The model under review builds one solid part; all positions refer to its coordinate system, in mm. Face numbers are marked on the shaded views. A direction names the side the tool comes from. Round coordinates to 2 decimals unless told otherwise and drop trailing zeros. Order: outer loops, then holes, each group sorted by start corner. A loop starts at its lowest first (then second) coordinate and runs counter-clockwise, first axis right, second up. Notation, with made-up numbers: M 27,-21.5 L 75,-21.5 A21 ccw 75,13.5 Z; hole C -3.75,85 d1. An arc over 180 degrees is marked long. Answer as a JSON object with one key per item and string values. Group by question number.
1. Add section D-D on y = -29.5. State the section outline as (x, z) points, and give its area (3 significant figures).
2. Clearance check with flat-ended pins moving along their axes: P1, Ø1, axis at y = -17, z = 6, coming from the +X side; P2, Ø16, axis at x = 0.5, y = -4, coming from the +Z side; P3, Ø1.5, axis at y = -32.5, z = 1, coming from the -X side; P4, Ø10, axis at x = 11, y = 0.5, coming from the -Z side. State where each tip first meets the part, or that it passes through.
3. Add section B-B on x = 8. State the section outline as (y, z) points, and give its area (3 significant figures).
4. To check wall thickness, follow probe 1 along Y at (x, z) = (0, 4); probe 2 along Y at (x, z) = (-2.5, 6.5); probe 3 along X at (y, z) = (-36, 7). State the ranges of each line that lie inside material, in increasing order. Write a range as [from, to].
5. Add section C-C on z = 1. State the section outline as (x, y) points.
6. Add section A-A on y = 4.5. State the section outline as (x, z) points.
7. Machinability: for the marked faces 4 and 5, which of the approach directions +Z, -Z, +X, -X, +Y, -Y give a long, thin tool a straight path to every point of the face, cutting with its end or side? Answer none if there is none.
8. Mouldability with a two-part tool opening along Y and no side actions: class the marked faces 1, 2 and 3 as released by +Y, released by -Y, zero draft, split by the parting line, or undercut.
```python
from build123d import *

# Parameters (mm, degrees)
SKETCH_R     = 16
SKETCH_R_2   = 11
PAD_DEPTH    = 7
SKETCH001_R  = 4
PAD001_DEPTH = 25


with BuildPart() as part:
    # Sketch → Pad (new body)
    with BuildSketch(Plane.XY):
        Circle(SKETCH_R)
        Circle(SKETCH_R_2, mode=Mode.SUBTRACT)
    extrude(amount=PAD_DEPTH)

    # Sketch001 → Pad001 (join)
    with BuildSketch(Plane.XZ.offset(14)):
        with Locations((0, 4)):
            Circle(SKETCH001_R)
    extrude(amount=PAD001_DEPTH)


solid = part.part
```
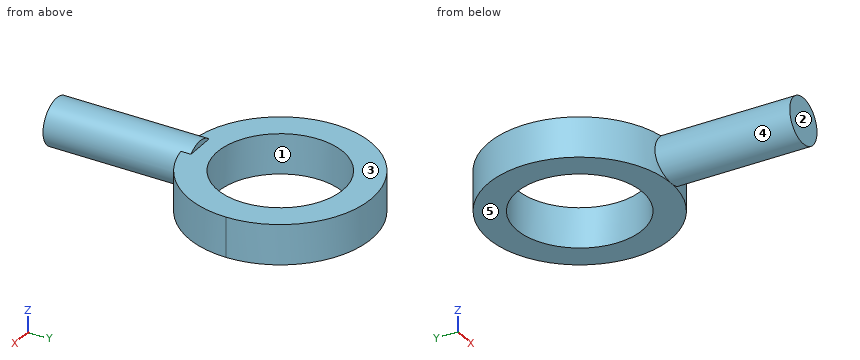
Recorded:
{
 "1": {"outline": "C 0,4 d8", "area": "50.3 mm²"},
 "2": {"P1": "stops at x = 3.71", "P2": "stops at z = 7", "P3": "stops at x = -3.31", "P4": "stops at z = 0"},
 "3": {"outline": "M -13.86,0 L -7.55,0 L -7.55,7 L -13.86,7 Z; M 7.55,0 L 13.86,0 L 13.86,7 L 7.55,7 Z", "area": "88.3 mm²"},
 "4": {"probe 1": "y = [-39, -11], [11, 16]", "probe 2": "y = [-39, -10.71], [10.71, 15.8]", "probe 3": "x = [-2.65, 2.65]"},
 "5": {"outline": "M -2.65,-39 L 2.65,-39 L 2.65,-15.78 A16 ccw long -2.65,-15.78 Z; hole C 0,0 d22"},
 "6": {"outline": "M -15.35,0 L -10.04,0 L -10.04,7 L -15.35,7 Z; M 10.04,0 L 15.35,0 L 15.35,7 L 10.04,7 Z"},
 "7": {"face 4": "-Y", "face 5": "-Z, +X, -X, +Y, -Y"},
 "8": {"face 1": "undercut", "face 2": "released by -Y", "face 3": "zero draft"}
}
